Can you work these out from the model? Positions are in its coordinate system, mm. A direction names the side the tool comes from. Round coordinates to 2 decimals unless told otherwise and drop trailing zeros. Loops run counter-clockwise (first coordinate to the right, second up) from the corner with the lowest first, then second, coordinate; pieces in that order, holes last.
(1) If I drill on line 1 along Z through (x, y) = (1.75, 2.25); line 2 along X through (y, z) = (7, -0.25); line 3 along X through (y, z) = (8.25, -8), over which ranges is the centre line in solid material (lowest first)?
(2) Will this pin go through, and if not, where does the flat tip stop? pin 1 Ø4 at (x, z) = (1, 10) entering from -Y.
(3) I want a section at A-A on z = 3.25. Write out the boundary of the cut face in (x, y), plus the area to 3 significant figures.
(4) Which directions (+Z, -Z, +X, -X, +Y, -Y) give clear straight access to the entire face, cutting with the end or side of a thin tool? Please do faces 4 (the face through (5, 0, 0)), 5 (the face through (7.4, 7, 0)), 6 (the face through (-2, 4, 7.5)), 7 (the face through (1, 10.9, 10)), 8 (the face through (0, 3.9, -10)).
(5) Thinking about a two-plate mould opening in Y: for faces 1 (the face through (-3.5, 7, 10)), 2 (the face through (-3.75, 7, 0)), 3 (the face through (5, 14.8, 0)), which applies, released by +Y, released by -Y, zero draft, split by the parting line, or undercut?
(6) I want a section at C-C on z = 11.25. Write out the boundary of the cut face in (x, y), plus the area to 3 significant figures.
(7) I want a section at D-D on x = 2.25. Write out the boundary of the cut face in (y, z).
(8) I want a section at B-B on y = 10.25. Write out the boundary of the cut face in (x, z), plus the area to 3 significant figures.
Autodesk Inventor part; units mm, degrees
ref_plane "YZ Plane" through (0, 0, 0) normal (1, 0, 0) x (0, 1, 0)
ref_plane "XZ Plane" through (0, 0, 0) normal (0, 1, 0) x (-1, 0, 0)
ref_plane "XY Plane" through (0, 0, 0) normal (0, 0, 1) x (1, 0, 0)
sketch "Sketch1" plane through (0, 0, 0) normal (0, 1, 0) x (-1, 0, 0)
  line L0 (7.4, 12.5) -> (-7.4, 12.5)
  line L1 (-7.4, 12.5) -> (-7.4, -12.5)
  line L2 (-7.4, -12.5) -> (7.4, -12.5)
  line L3 (7.4, -12.5) -> (7.4, 12.5)
  line L4 (3.75, 7.5) -> (-3.75, 7.5)
  line L5 (-3.75, 7.5) -> (-3.75, -7.5)
  line L6 (-3.75, -7.5) -> (3.75, -7.5)
  line L7 (3.75, -7.5) -> (3.75, 7.5)
  point P0 (0, 0)
  dimension "d0" = 14.8
  dimension "d1" = 25
  dimension "d2" = 12.5
  dimension "d3" = 7.4
  dimension "d4" = 7.5
  dimension "d5" = 15
  dimension "d6" = 3.75
  dimension "d7" = 7.5
extrude "Extrusion1" add sketch "Sketch1" along normal blind 14.8
sketch "Sketch2" plane through (-7.4, 0, 12.5) normal (0, 0, 1) x (1, 0, 0)
  line L0 (3.9, 10.9) -> (10.9, 10.9)
  line L1 (10.9, 10.9) -> (10.9, 3.9)
  line L2 (10.9, 3.9) -> (3.9, 3.9)
  line L3 (3.9, 3.9) -> (3.9, 10.9)
  line L4 (0, 0) -> (14.8, 0)
  line L5 (14.8, 0) -> (14.8, 14.8)
  point P0 (7.4, 0)
  point P1 (7.4, 0)
  point P2 (7.4, 3.9)
  point P3 (14.8, 7.4)
  point P4 (10.9, 7.4)
  dimension "d10" = 7
  dimension "d11" = 7
  dimension "d12" = 0
  dimension "d13" = 0
extrude "Extrusion2" cut sketch "Sketch2" against normal through all
chamfer "Chamfer1" distance 2 angle 45 7 edges at (-3.5, 10.9, 10) (-3.5, 3.9, 10) (3.5, 3.9, 10) (-3.5, 3.9, -10) (3.5, 3.9, -10) (3.5, 10.9, -10) (-3.5, 10.9, -10)
chamfer "Chamfer2" distance 0.5 angle 45 4 edges at (7.4, 0, 0) (7.4, 14.8, 0) (-7.4, 14.8, 0) (-7.4, 0, 0)
properties part number "Test Square"
Filled sheet:
1. line 1: z = -12.5 to -7.5, 7.5 to 12.5
1. line 2: x = -7.4 to -3.75, 3.75 to 7.4
1. line 3: x = -7.4 to -3.5, 3.5 to 7.4
2. pin 1: stops at y = 0
3. outline: (-7.4, 0.5) - (-6.9, 0) - (-3.75, 0) - (-3.75, 14.8) - (-6.9, 14.8) - (-7.4, 14.3) - close; (3.75, 0) - (6.9, 0) - (7.4, 0.5) - (7.4, 14.3) - (6.9, 14.8) - (3.75, 14.8) - close
3. area: 108 mm2
4. face 4: +Z, -Z, +X, -X, -Y
4. face 5: +Z, -Z, +X, +Y, -Y
4. face 6: +Y, -Y
4. face 7: +Z
4. face 8: +Z, -Z
5. face 1: undercut
5. face 2: zero draft
5. face 3: released by +Y
6. outline: (-7.4, 0.5) - (-6.9, 0) - (6.9, 0) - (7.4, 0.5) - (7.4, 14.3) - (6.9, 14.8) - (-6.9, 14.8) - (-7.4, 14.3) - close; hole (-3.5, 5.9) - (-1.5, 3.9) - (1.5, 3.9) - (3.5, 5.9) - (3.5, 10.9) - (-1.5, 10.9) - (-3.5, 8.9) - close
6. area: 176 mm2
7. outline: (0, -12.5) - (4.65, -12.5) - (4.65, -7.5) - (0, -7.5) - close; (0, 7.5) - (4.65, 7.5) - (4.65, 12.5) - (0, 12.5) - close; (10.15, -12.5) - (14.8, -12.5) - (14.8, -7.5) - (10.15, -7.5) - close; (10.9, 7.5) - (14.8, 7.5) - (14.8, 12.5) - (10.9, 12.5) - close
8. outline: (-7.4, -12.5) - (-2.15, -12.5) - (-2.15, -7.5) - (-3.75, -7.5) - (-3.75, 7.5) - (-2.15, 7.5) - (-2.15, 12.5) - (-7.4, 12.5) - close; (2.15, -12.5) - (7.4, -12.5) - (7.4, 12.5) - (3.5, 12.5) - (3.5, 7.5) - (3.75, 7.5) - (3.75, -7.5) - (2.15, -7.5) - close
8. area: 208 mm2
